The model under review builds one solid part; all positions refer to its coordinate system, in mm. Coordinates: 2 decimals unless noted, no trailing zeros. Write each loop counter-clockwise with the first axis right and the second up, starting at its lowest first coordinate (ties: lowest second). Pieces come first, ordered by that corner, then holes. Notation, with made-up numbers: M 73.5,-4 L 89.5,-4 A15 cw 89.5,0 Z; hole C -29,24 d6. An arc over 180 degrees is marked long. Answer as a JSON object with one key per item and string values.
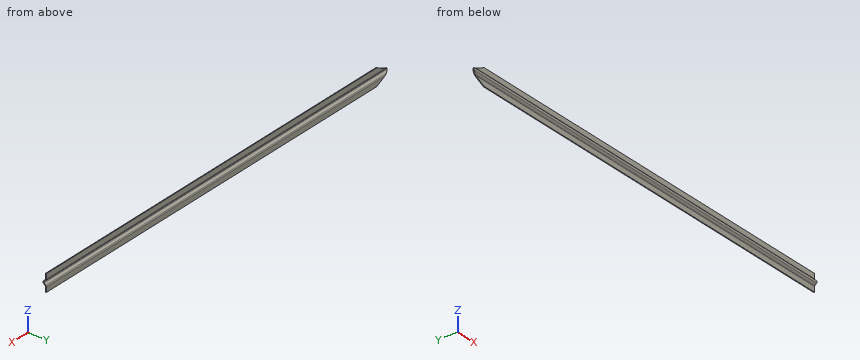
```python
from build123d import *

# Parameters (mm, degrees)
SHEET_EXTRUDE_1_1_BACK   = 500
SHEET_EXTRUDE_1_1_DEPTH  = 1000
THICKEN_1_T1             = 1
THICKEN_1_T2             = 1
FILLET_1_R               = 2
FILLET_2_R               = 4
CUT_EXTRUDE_1_DEPTH      = 501.445463467
CUT_EXTRUDE_1_DEPTH_BACK = 501.445463467


with BuildPart() as body_1:
    # Sheet Extrude 1: a surface, the sketch's curves swept straight by 1000 mm
    with BuildLine(Plane(origin=(0, 0, 0), x_dir=(0, 0, -1), z_dir=(1, 0, 0)).offset(-SHEET_EXTRUDE_1_1_BACK), mode=Mode.PRIVATE) as sheet_extrude_1_1_path:
        Line((-20, 0), (-7, 0))
        Line((-7, 0), (0, -7))
        Line((0, -7), (7, 0))
        Line((7, 0), (20, 0))
    sheet_extrude_1_1 = Shell.extrude(sheet_extrude_1_1_path.wire(), (1 * SHEET_EXTRUDE_1_1_DEPTH, 0 * SHEET_EXTRUDE_1_1_DEPTH, 0 * SHEET_EXTRUDE_1_1_DEPTH))
    add(Solid.thicken(sheet_extrude_1_1, THICKEN_1_T1))
    add(Solid.thicken(sheet_extrude_1_1, -THICKEN_1_T2))

    # Скругление1
    fillet_1_edges = [body_1.edges().sort_by_distance(p)[0] for p in [
        (0, -5.585786438, 0),
        (0, -1, -7.414213562),
        (0, -1, 7.414213562),
    ]]
    fillet(fillet_1_edges, radius=FILLET_1_R)

    # Скругление2
    fillet_2_edges = [body_1.edges().sort_by_distance(p)[0] for p in [
        (0, 1, 6.585786438),
        (0, 1, -6.585786438),
        (0, -8.414213562, 0),
    ]]
    fillet(fillet_2_edges, radius=FILLET_2_R)

    # Эскиз2 → Вырез-Вытянуть1 (cut, two sides: drawn at the far end of the back side and taken through both)
    with BuildSketch(Plane(origin=(0, 0, 0), x_dir=(1, 0, 0), z_dir=(0, 1, 0)).offset(-CUT_EXTRUDE_1_DEPTH_BACK)):
        with BuildLine():
            Line((1267.734544165, -883.867272083), (-460, -20))
            Line((-460, -20), (-494.633436854, -2.683281573))
            ThreePointArc((-494.633436854, -2.683281573), (-496.291796068, 0), (-494.633436854, 2.683281573))
            Line((-494.633436854, 2.683281573), (-460, 20))
            Line((-460, 20), (1267.734544165, 883.867272083))
            Line((1267.734544165, 883.867272083), (-2595.597343663, 883.867272083))
            Line((-2595.597343663, 883.867272083), (-2595.597343663, -883.867272083))
            Line((-2595.597343663, -883.867272083), (1267.734544165, -883.867272083))
        make_face()
    extrude(amount=CUT_EXTRUDE_1_DEPTH + CUT_EXTRUDE_1_DEPTH_BACK, mode=Mode.SUBTRACT)


solid = body_1.part
```
(1) Wall thickness on line 1 along Z through (x, y) = (-49, -3); line 2 along Y through (x, z) = (-150.5, -12.5); line 3 along Z through (x, y) = (-313.5, -5.75): over which ranges is each line inside the solid? List them lowest first. Write a range as from..to.
Results list:
{"line 1": "-5.41..-2.59, 2.59..5.41", "line 2": "-1..1", "line 3": "-2.65..2.65"}
(2) For pin 1 Ø3 at (x, z) = (-62, -3.5) entering from -Y; pin 2 Ø6 at (x, z) = (231.5, -14.5) entering from -Y; pin 3 Ø2 at (x, z) = (-286, -8.5) entering from -Y, all flat-tipped, find the tip position at first contact; note any pin that passes through.
Results list:
{"pin 1": "y = -6.22", "pin 2": "y = -1", "pin 3": "y = -1.14"}
(3) Add section A-A on x = -180. Give the boundary of the cut face in (y, z), and give its area (3 significant figures).
Results list:
{"outline": "M -5.59,-2.83 L -1.59,-6.83 A2 cw -1,-8.24 L -1,-20 L 1,-20 L 1,-8.24 A4 ccw -0.17,-5.41 L -4.17,-1.41 A2 cw -4.17,1.41 L -0.17,5.41 A4 ccw 1,8.24 L 1,20 L -1,20 L -1,8.24 A2 cw -1.59,6.83 L -5.59,2.83 A4 ccw Z", "area": "88.5 mm²"}
